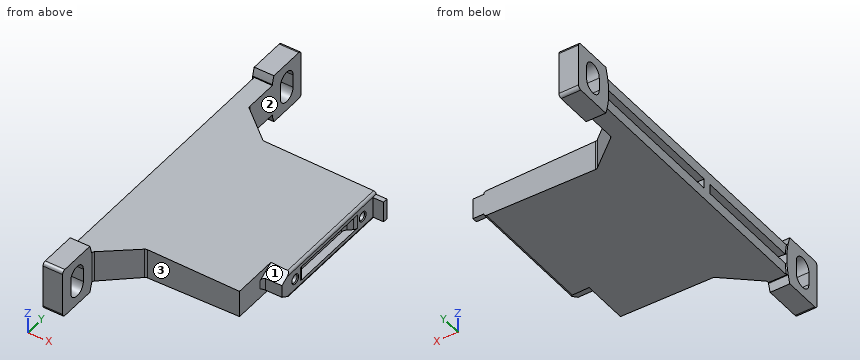
```python
from build123d import *

# Parameters (mm, degrees)
BOSS_EXTRUDE1_DEPTH      = 51
CUT_EXTRUDE1_DEPTH       = 10
CUT_EXTRUDE1_DEPTH_BACK  = 10
CUT_EXTRUDE2_DEPTH       = 10
CUT_EXTRUDE2_DEPTH_BACK  = 10
CUT_EXTRUDE3_DEPTH       = 10
CUT_EXTRUDE3_DEPTH_BACK  = 10
CUT_EXTRUDE4_DEPTH       = 0.5
CUT_EXTRUDE4_DEPTH_BACK  = 0.5
CUT_EXTRUDE5_DEPTH       = 80.4
CUT_EXTRUDE6_DEPTH       = 1.5
CUT_EXTRUDE6_DEPTH_BACK  = 1.5
SKETCH8_W                = 3.8
SKETCH8_H                = 1.5
BOSS_EXTRUDE2_DEPTH      = 3.2
BOSS_EXTRUDE2_DEPTH_BACK = 3.2
CUT_EXTRUDE7_DEPTH       = 2.15
CUT_EXTRUDE7_DEPTH_BACK  = 2.15
CUT_EXTRUDE8_DEPTH       = 6
CUT_EXTRUDE8_DEPTH_BACK  = 6


with BuildPart() as part:
    # Sketch1 → Boss-Extrude1 (new body)
    with BuildSketch(Plane(origin=(0, 0, 0), x_dir=(0, 0, -1), z_dir=(1, 0, 0))):
        with BuildLine():
            Line((-7.5, 105), (-7.5, 93.91788212))
            ThreePointArc((-7.5, 93.91788212), (-6.261006558, 93.509722693), (-5, 93.175714714))
            Line((-5, 93.175714714), (-5, 12.824285286))
            ThreePointArc((-5, 12.824285286), (-6.261006558, 12.490277307), (-7.5, 12.08211788))
            Line((-7.5, 12.08211788), (-7.5, 1))
            ThreePointArc((-7.5, 1), (-7.207106781, 0.292893219), (-6.5, 0))
            Line((-6.5, 0), (6.5, 0))
            ThreePointArc((6.5, 0), (7.207106781, 0.292893219), (7.5, 1))
            Line((7.5, 1), (7.5, 12.08211788))
            ThreePointArc((7.5, 12.08211788), (6.261006558, 12.490277307), (5, 12.824285286))
            Line((5, 12.824285286), (5, 93.175714714))
            ThreePointArc((5, 93.175714714), (6.261006558, 93.509722693), (7.5, 93.91788212))
            Line((7.5, 93.91788212), (7.5, 105))
            ThreePointArc((7.5, 105), (7.207106781, 105.707106781), (6.5, 106))
            Line((6.5, 106), (-6.5, 106))
            ThreePointArc((-6.5, 106), (-7.207106781, 105.707106781), (-7.5, 105))
        make_face()
    extrude(amount=BOSS_EXTRUDE1_DEPTH)

    # Sketch2 → Cut-Extrude1 (cut, two sides)
    with BuildSketch(Plane.XY) as cut_extrude1_sk:
        with BuildLine():
            Line((6, 155.065), (6, 83.209033859))
            ThreePointArc((6, 83.209033859), (6.093692213, 82.786415598), (6.35721239, 82.442989416))
            Line((6.35721239, 82.442989416), (16.021182625, 74.333955557))
            ThreePointArc((16.021182625, 74.333955557), (16.321950091, 74.160307379), (16.663970234, 74.1))
            Line((16.663970234, 74.1), (95, 74.1))
            Line((95, 74.1), (95, 32.2))
            Line((95, 32.2), (45.8, 32.2))
            ThreePointArc((45.8, 32.2), (45.092893219, 31.907106781), (44.8, 31.2))
            Line((44.8, 31.2), (44.8, 22.1))
            Line((44.8, 22.1), (16.663970234, 22.1))
            ThreePointArc((16.663970234, 22.1), (16.321950091, 22.039692621), (16.021182625, 21.866044443))
            Line((16.021182625, 21.866044443), (6.285769912, 13.697063227))
            ThreePointArc((6.285769912, 13.697063227), (6.07495377, 13.422322282), (6, 13.084227672))
            Line((6, 13.084227672), (6, -150))
            Line((6, -150), (100, -150))
            Line((100, -150), (100, 155.065))
            Line((100, 155.065), (6, 155.065))
        make_face()
    extrude(amount=CUT_EXTRUDE1_DEPTH, mode=Mode.SUBTRACT)
    extrude(cut_extrude1_sk.sketch, amount=-CUT_EXTRUDE1_DEPTH_BACK, mode=Mode.SUBTRACT)

    # Sketch3 → Cut-Extrude2 (cut, two sides)
    with BuildSketch(Plane(origin=(0, 0, 0), x_dir=(0, 0, -1), z_dir=(1, 0, 0))) as cut_extrude2_sk:
        with BuildLine():
            Line((-2, 3.6), (2, 3.6))
            ThreePointArc((2, 3.6), (4.799999867, 6.4), (2, 9.2))
            Line((2, 9.2), (-2, 9.2))
            ThreePointArc((-2, 9.2), (-4.799999867, 6.4), (-2, 3.6))
        make_face()
    extrude(amount=CUT_EXTRUDE2_DEPTH, mode=Mode.SUBTRACT)
    extrude(cut_extrude2_sk.sketch, amount=-CUT_EXTRUDE2_DEPTH_BACK, mode=Mode.SUBTRACT)

    # Sketch4 → Cut-Extrude3 (cut, two sides)
    with BuildSketch(Plane(origin=(0, 0, 0), x_dir=(0, 0, -1), z_dir=(1, 0, 0))) as cut_extrude3_sk:
        with BuildLine():
            Line((-2, 96.8), (2, 96.8))
            ThreePointArc((2, 96.8), (4.799999867, 99.6), (2, 102.4))
            Line((2, 102.4), (-2, 102.4))
            ThreePointArc((-2, 102.4), (-4.799999867, 99.6), (-2, 96.8))
        make_face()
    extrude(amount=CUT_EXTRUDE3_DEPTH, mode=Mode.SUBTRACT)
    extrude(cut_extrude3_sk.sketch, amount=-CUT_EXTRUDE3_DEPTH_BACK, mode=Mode.SUBTRACT)

    # Sketch5 → Cut-Extrude4 (cut, two sides)
    with BuildSketch(Plane(origin=(0, 0, 0), x_dir=(0, 0, -1), z_dir=(1, 0, 0))) as cut_extrude4_sk:
        with BuildLine():
            Line((-8, 94.106098468), (-8, 11.893901532))
            ThreePointArc((-8, 11.893901532), (0, 13.4), (8, 11.893901532))
            Line((8, 11.893901532), (8, 94.106098468))
            ThreePointArc((8, 94.106098468), (0, 92.6), (-8, 94.106098468))
        make_face()
    extrude(amount=CUT_EXTRUDE4_DEPTH, mode=Mode.SUBTRACT)
    extrude(cut_extrude4_sk.sketch, amount=-CUT_EXTRUDE4_DEPTH_BACK, mode=Mode.SUBTRACT)

    # Sketch6 → Cut-Extrude5 (cut)
    with BuildSketch(Plane(origin=(0, 12.8, 0), x_dir=(1, 0, 0), z_dir=(0, 1, 0))):
        with BuildLine():
            Line((-7.83333, -20.4458), (56.7096, -20.4458))
            Line((56.7096, -20.4458), (56.7096, 14.6041))
            Line((56.7096, 14.6041), (-7.83333, 14.6041))
            Line((-7.83333, 14.6041), (-7.83333, 5.029470245))
            Line((-7.83333, 5.029470245), (50.013961925, 4.019742008))
            ThreePointArc((50.013961925, 4.019742008), (50.570600359, 3.780591263), (50.8, 3.219863852))
            Line((50.8, 3.219863852), (50.8, -3.219863852))
            ThreePointArc((50.8, -3.219863852), (50.570600359, -3.780591263), (50.013961925, -4.019742008))
            Line((50.013961925, -4.019742008), (-7.83333, -5.029470245))
            Line((-7.83333, -5.029470245), (-7.83333, -20.4458))
        make_face()
    extrude(amount=CUT_EXTRUDE5_DEPTH, mode=Mode.SUBTRACT)

    # Sketch7 → Cut-Extrude6 (cut, two sides)
    with BuildSketch(Plane.XY) as cut_extrude6_sk:
        with BuildLine():
            Line((-49.796416348, 97.062832237), (-49.796416348, 8.937167763))
            Line((-49.796416348, 8.937167763), (3.5, 13.6))
            Line((3.5, 13.6), (14.898143221, 23.164177772))
            ThreePointArc((14.898143221, 23.164177772), (16.101213086, 23.858770483), (17.469293659, 24.1))
            Line((17.469293659, 24.1), (40.8, 24.1))
            ThreePointArc((40.8, 24.1), (42.214213562, 24.685786438), (42.8, 26.1))
            Line((42.8, 26.1), (42.8, 32.2))
            ThreePointArc((42.8, 32.2), (43.385786438, 33.614213562), (44.8, 34.2))
            Line((44.8, 34.2), (45.3, 34.2))
            ThreePointArc((45.3, 34.2), (45.653553391, 34.346446609), (45.8, 34.7))
            Line((45.8, 34.7), (45.8, 42.907575802))
            ThreePointArc((45.8, 42.907575802), (45.244727924, 44.290601913), (43.887238775, 44.905672245))
            Line((43.887238775, 44.905672245), (-0.5, 46.843660943))
            Line((-0.5, 46.843660943), (-0.5, 49.356339057))
            Line((-0.5, 49.356339057), (43.887238775, 51.294327755))
            ThreePointArc((43.887238775, 51.294327755), (45.244727924, 51.909398087), (45.8, 53.292424198))
            Line((45.8, 53.292424198), (45.8, 70.1))
            ThreePointArc((45.8, 70.1), (45.214213562, 71.514213562), (43.8, 72.1))
            Line((43.8, 72.1), (16.396715426, 72.1))
            ThreePointArc((16.396715426, 72.1), (15.028634853, 72.341229517), (13.825564987, 73.035822228))
            Line((13.825564987, 73.035822228), (3.5, 81.7))
            Line((3.5, 81.7), (3.5, 92.4))
            Line((3.5, 92.4), (-49.796416348, 97.062832237))
        make_face()
    extrude(amount=CUT_EXTRUDE6_DEPTH, mode=Mode.SUBTRACT)
    extrude(cut_extrude6_sk.sketch, amount=-CUT_EXTRUDE6_DEPTH_BACK, mode=Mode.SUBTRACT)

    # Sketch8 → Boss-Extrude2 (add, two sides)
    with BuildSketch(Plane.XY) as boss_extrude2_sk:
        with Locations((52.2, 73.35)):
            Rectangle(SKETCH8_W, SKETCH8_H)
    extrude(amount=BOSS_EXTRUDE2_DEPTH)
    extrude(boss_extrude2_sk.sketch, amount=-BOSS_EXTRUDE2_DEPTH_BACK)

    # Sketch9 → Cut-Extrude7 (cut, two sides)
    with BuildSketch(Plane.XY) as cut_extrude7_sk:
        with BuildLine():
            Line((48.4, 62.270122483), (48.4, 43.929877517))
            ThreePointArc((48.4, 43.929877517), (48.563961373, 43.190295559), (49.025121683, 42.589299741))
            Line((49.025121683, 42.589299741), (50.335623893, 41.48965782))
            ThreePointArc((50.335623893, 41.48965782), (50.678200123, 41.043203785), (50.8, 40.493800044))
            Line((50.8, 40.493800044), (55.7133, 36.977251782))
            Line((55.7133, 36.977251782), (55.7133, 69.222748218))
            Line((55.7133, 69.222748218), (50.8, 65.706199956))
            ThreePointArc((50.8, 65.706199956), (50.678200123, 65.156796215), (50.335623893, 64.71034218))
            Line((50.335623893, 64.71034218), (49.025121683, 63.610700259))
            ThreePointArc((49.025121683, 63.610700259), (48.563961373, 63.009704441), (48.4, 62.270122483))
        make_face()
    extrude(amount=CUT_EXTRUDE7_DEPTH, mode=Mode.SUBTRACT)
    extrude(cut_extrude7_sk.sketch, amount=-CUT_EXTRUDE7_DEPTH_BACK, mode=Mode.SUBTRACT)

    # Sketch10 → Cut-Revolve1 (revolve, cut)
    with BuildSketch(Plane.XY):
        Polygon((45.8, 68.1), (45.8, 69.6), (46.0705, 69.3295), (50.5295, 69.3295), (50.8, 69.6), (50.8, 68.1), align=None)
    revolve(axis=Axis((50.8, 68.1, 0), (-1, 0, 0)), mode=Mode.SUBTRACT)

    # Sketch11 → Cut-Revolve2 (revolve, cut)
    with BuildSketch(Plane.XY):
        Polygon((45.8, 38.1), (45.8, 39.6), (46.0705, 39.3295), (50.5295, 39.3295), (50.8, 39.6), (50.8, 38.1), align=None)
    revolve(axis=Axis((50.8, 38.1, 0), (-1, 0, 0)), mode=Mode.SUBTRACT)

    # Sketch12 → Cut-Extrude8 (cut, two sides)
    with BuildSketch(Plane(origin=(50.8, 0, 0), x_dir=(0, 0, -1), z_dir=(1, 0, 0))) as cut_extrude8_sk:
        Polygon((-16.0833, 30.7), (16.9167, 30.7), (16.9167, 58.209687362), (1.322649731, 31.2), (-1.322649731, 31.2), (-16.0833, 56.766196219), align=None)
    extrude(amount=CUT_EXTRUDE8_DEPTH, mode=Mode.SUBTRACT)
    extrude(cut_extrude8_sk.sketch, amount=-CUT_EXTRUDE8_DEPTH_BACK, mode=Mode.SUBTRACT)


solid = part.part
```
CAD build for the part. Positions are in the model's coordinates, mm. Face numbers are marked on the shaded views. A direction names the side the tool comes from. Coordinates: 2 decimals unless noted, no trailing zeros. Order: outer loops, then holes, each group sorted by start corner. A loop starts at its lowest first (then second) coordinate and runs counter-clockwise, first axis right, second up. Notation, with made-up numbers: (13.25, -13) - (17.25, -13) arc R14 ccw to (17.25, 1) - close; hole circle Ø10 at (22, -31.75). An arc over 180 degrees is marked (long way). Use a Markdown table: item, result. Add a question column.
(1) Saw through at C-C (y = 18.5). Give the cut face in (x, z).
(2) Drill centre lines: line 1 along Y through (x, z) = (47.2, 0); line 2 along Z through (x, y) = (49, 51.5); line 3 along Z through (x, y) = (48.6, 68.1). Where is each one in solid material? Low to high. Write a range as [from, to].
(3) Which spindle directions (+Z, -Z, +X, -X, +Y, -Y) get a long thin tool onto all of the face, cutting with end or side? Do the marked faces 1, 2 and 3. Say none if no direction does.
(4) Flat gauge pins, fed straight in: pin 1 (13 mm diameter, centred on x = 13.5, y = 67, fed in from -Z); pin 2 (3 mm diameter, centred on x = 16.5, z = -3.5, fed in from -Y); pin 3 (6.5 mm diameter, centred on y = 31, z = -1, fed in from +X); pin 4 (8 mm diameter, centred on y = 17, z = -0.5, fed in from -X). Where does each tip first touch, or does it go through?
(5) Saw through at D-D (x = 26). Give the cut face in (y, z), then the cut area to 3 significant figures.
(6) Saw through at A-A (y = 6.4). Give the cut face in (x, z).
(7) Saw through at B-B (x = 39). Give the cut face in (y, z).
Solved:
| question | item | result |
|---|---|---|
| 1 | outline | (0.5, -4.88) - (12.01, -4.68) - (12.01, 4.68) - (0.5, 4.88) - (0.5, 1.5) - (9.34, 1.5) - (9.34, -1.5) - (0.5, -1.5) - close |
| 2 | line 1 | y = [32.2, 36.87], [39.33, 66.87], [69.33, 74.1] |
| 2 | line 2 | z = [-4.04, -2.15], [2.15, 4.04] |
| 2 | line 3 | z = [-4.04, -1.23], [1.23, 4.04] |
| 3 | face 1 | +Z, +X, -Y |
| 3 | face 2 | +Z, -Z, +X, +Y |
| 3 | face 3 | +Z, -Z, +X, -Y |
| 4 | pin 1 | stops at z = -4.77 |
| 4 | pin 2 | stops at y = 21.01 |
| 4 | pin 3 | stops at x = 50.8 |
| 4 | pin 4 | stops at x = 0 |
| 5 | outline | (22.1, -4.44) - (74.1, -4.44) - (74.1, 4.44) - (22.1, 4.44) - close; hole (24.1, -1.5) - (45.69, -1.5) - (45.69, 1.5) - (24.1, 1.5) - close; hole (50.51, -1.5) - (72.1, -1.5) - (72.1, 1.5) - (50.51, 1.5) - close |
| 5 | area | 332 mm² |
| 6 | outline | (0, -7.5) - (6, -7.5) - (6, -4.8) - (0, -4.8) - close; (0, 4.8) - (6, 4.8) - (6, 7.5) - (0, 7.5) - close |
| 7 | outline | (22.1, -4.21) - (74.1, -4.21) - (74.1, 4.21) - (22.1, 4.21) - close; hole (24.1, -1.5) - (45.12, -1.5) - (45.12, 1.5) - (24.1, 1.5) - close; hole (51.08, -1.5) - (72.1, -1.5) - (72.1, 1.5) - (51.08, 1.5) - close |
